Source: CAD feature listing. Evaluate the final solid. Frame: model axes, mm. A direction names the side the tool comes from. Give positions to 0.01 mm unless a question says otherwise; leave off trailing zeros. Order: outer loops, then holes, each group sorted by start corner. A loop starts at its lowest first (then second) coordinate and runs counter-clockwise, first axis right, second up. Notation, with made-up numbers: (54.5, -37.75) - (109.5, -37.75) arc R9 cw to (109.5, -26.75) - close; hole circle Ø5 at (51, 36). An arc over 180 degrees is marked (long way). Answer as CSV lines item,"result".
```python
from build123d import *

# Parameters (mm, degrees)
F1_DEPTH = 47
F3_D     = 7
F4_W     = 54
F4_H     = 30
F5_DEPTH = 40.001
F6_R     = 9.99999
F8_R     = 5
F10_D    = 4.5
F11_SIZE = 5


# Not quite as in the source:
# - a fillet or chamfer is up to 0.001 mm smaller than in the source, because OpenCascade refuses the exact size


with BuildPart() as f1:
    # F0 (on Front) → F1 (new body)
    with BuildSketch(Plane.XZ):
        Polygon((27, 40), (-27, 40), (-27, 30), (-10, 30), (-10, -25), (10, -25), (10, 30), (27, 30), align=None)
    extrude(amount=F1_DEPTH)

    # F3 (through all)
    with Locations(Plane(origin=(0, 0, -25), x_dir=(1, 0, 0), z_dir=(0, 0, -1))):
        with Locations((0, 37)):
            Hole(F3_D / 2)

    # F4 (on Top) → F5 (cut, through all)
    with BuildSketch(Plane.XY):
        with Locations((0, -32)):
            Rectangle(F4_W, F4_H)
    extrude(amount=F5_DEPTH, mode=Mode.SUBTRACT)

    # F6 (radius 10 in the source; OpenCascade refuses exactly that, so slightly less here)
    f6_edges = [f1.edges().sort_by_distance(p)[0] for p in [
        (-10, -47, -12.5),
        (10, -47, -12.5),
    ]]
    fillet(f6_edges, radius=F6_R)

    # F8
    f8_edges = [f1.edges().sort_by_distance(p)[0] for p in [
        (10, -8.5, 30),
        (-10, -8.5, 30),
    ]]
    fillet(f8_edges, radius=F8_R)

    # F10 (through all)
    with Locations(Plane.XY.offset(40)):
        with Locations((-20, -8.5), (20, -8.5)):
            Hole(F10_D / 2)

    # F11
    f11_edges = [f1.edges().sort_by_distance(p)[0] for p in [
        (0, -17, 0),
    ]]
    chamfer(f11_edges, length=F11_SIZE)


solid = f1.part
```
(1) Cut plane B-B (x = -20). Return loops of the section in (y, z), then the cut area to 3 significant figures.
Completed:
outline,"(-17, 30) - (-10.75, 30) - (-10.75, 40) - (-17, 40) - close; (-6.25, 30) - (0, 30) - (0, 40) - (-6.25, 40) - close"
area,"125 mm²"
(2) Cut plane A-A (y = -8.5). Return loops of the section in (x, z), then the cut area to 3 significant figures.
Completed:
outline,"(-27, 30) - (-22.25, 30) - (-22.25, 40) - (-27, 40) - close; (-17.75, 30) - (-15, 30) arc R5 cw to (-10, 25) - (-10, -25) - (10, -25) - (10, 25) arc R5 cw to (15, 30) - (17.75, 30) - (17.75, 40) - (-17.75, 40) - close; (22.25, 30) - (27, 30) - (27, 40) - (22.25, 40) - close"
area,"1,560 mm²"
(3) Access query for faces 1 (the flat face through (0, -17, 26)), 2 (the flat face through (22, -6, 30)), 3 (the flat face through (-10, -14, -5)). Directions: +Z, -Z, +X, -X, +Y, -Y. A direction counts if a zero-diameter tool reaches every point of the face in a straight line with its end or side. Return the directions, or none.
Completed:
face 1,"+Z, +X, -X, -Y"
face 2,"-Z, +X, +Y, -Y"
face 3,"-Z, -X, +Y, -Y"
(4) Ray query, line 1 (Y direction, x = 0, z = -13); line 2 (Y direction, x = -20, z = 36.25); line 3 (X direction, y = -8, z = 36). Return the intervals inside material, ascending. Write a range as from..to.
Completed:
line 1,"-47..-40.5, -33.5..0"
line 2,"-17..-10.75, -6.25..0"
line 3,"-27..-22.19, -17.81..17.81, 22.19..27"
(5) Contact query for flat-ended pins moving along their axis: pin 1 (13 mm diameter, centred on x = -21.5, y = -7, fed in from -Z); pin 2 (2 mm diameter, centred on y = -22, z = -4.5, fed in from -X); pin 3 (10.5 mm diameter, centred on x = 10.5, z = 16.5, fed in from -Y). Output: stop coordinate, or through.
Completed:
pin 1,"z = 30"
pin 2,"x = -10"
pin 3,"y = -17"
(6) Cut plane D-D (y = -35.5). Return loops of the section in (x, z), then the cut area to 3 significant figures.
Completed:
outline,"(-10, -25) - (-3.16, -25) - (-3.16, 0) - (-10, 0) - close; (3.16, -25) - (10, -25) - (10, 0) - (3.16, 0) - close"
area,"342 mm²"
(7) Mould query, pull axis Y, two halves, no side actions, for faces 4 (the cylindrical face through (0.46, -40.47, -12.33)), 5 (the cylindrical face through (7.15, -43.99, -12.32)), 6 (the flat face through (0, -32, 0)). Classes: released by +Y, released by -Y, zero draft, split by the parting line, or undercut.
Completed:
face 4,"undercut"
face 5,"released by -Y"
face 6,"zero draft"
